from build123d import *

# Parameters (mm, degrees)
F1_DEPTH = 10
F3_START = -1.5
F3_DEPTH = 7
F4_R     = 5


with BuildPart() as f1:
    # F0 (on Top) → F1 (new body)
    with BuildSketch(Plane.XY):
        Polygon((0, 18.8854382), (-29.0617011202, 40), (-17.9611190632, 5.83592135), align=None)
        Polygon((17.9611190632, 5.83592135), (29.0617011202, 40), (0, 18.8854382), align=None)
        Polygon((0, 18.8854382), (-17.9611190632, 5.83592135), (-11.100582057, -15.27864045), (11.100582057, -15.27864045), (17.9611190632, 5.83592135), align=None)
        Polygon((11.100582057, -15.27864045), (47.0228201834, -15.27864045), (17.9611190632, 5.83592135), align=None)
        Polygon((-11.100582057, -15.27864045), (0, -49.4427191), (11.100582057, -15.27864045), align=None)
        Polygon((-17.9611190632, 5.83592135), (-47.0228201834, -15.27864045), (-11.100582057, -15.27864045), align=None)
    extrude(amount=F1_DEPTH)

    # F2 (on face) → F3 (cut)
    with BuildSketch(Plane.XY.offset(10).offset(F3_START)):
        Polygon((-9.25, -11.1145618), (0, -11.1145618), (9.25, -11.1145618), (9.25, 25.605956584), (0, 18.8854382), (-9.25, 25.605956584), align=None)
    extrude(amount=-F3_DEPTH, mode=Mode.SUBTRACT)

    # F4
    f4_edges = [f1.edges().sort_by_distance(p)[0] for p in [
        (-17.961119, 5.835921, 5),
        (-11.100582, -15.27864, 5),
        (11.100582, -15.27864, 5),
        (17.961119, 5.835921, 5),
        (0, 18.885438, 9.25),
        (0, 18.885438, 0.75),
        (9.25, 25.605957, 5),
        (-9.25, 25.605957, 5),
    ]]
    fillet(f4_edges, radius=F4_R)


solid = f1.part
Could you check a few things on this model? Use its own coordinates, in mm. A direction names the side the tool comes from. Give positions to 0.01 mm unless a question says otherwise; leave off trailing zeros. Order: outer loops, then holes, each group sorted by start corner. A loop starts at its lowest first (then second) coordinate and runs counter-clockwise, first axis right, second up. Notation, with made-up numbers: (-15, -37.5) -> (17, -37.5) arc R31 ccw to (17, -4.5) -> close; hole circle Ø9 at (28.25, 40.5). An arc over 180 degrees is marked (long way). Answer in a Markdown table with one row per item. Add a question column.
Item 1: Imagine slicing it at C-C (y = -10). List the corners of the cut face in (x, z) for me, and give its area (3 significant figures).
Item 2: Please list where these lines run through material, in increasing order: probe 1 along Z at (x, y) = (8.5, 10); probe 2 along X at (y, z) = (7, 3); probe 3 along X at (y, z) = (-3, 6).
Item 3: We'd pull the mould along Y, two halves only. Please class faces 6 (the flat face through (31, -15.279, 5)), 7 (the flat face through (3, -1, 10)), 8 (the flat face through (-33.779, -5.656, 4.93)): pulls with the +Y half, pulls with the -Y half, needs draft (parallel to the pull), parting line crosses it, or undercut.
Item 4: Imagine slicing it at A-A (x = -25.5). List the corners of the cut face in (y, z) for me, and give its area (3 significant figures).
Item 5: Imagine slicing it at D-D (x = -7). List the corners of the cut face in (y, z) for me, and give its area (3 significant figures).
Item 6: I'm going to push flat-ended pins straight in: P1, Ø5.5, axis at y = 4.5, z = 6.5, coming from the +X side; P2, Ø3, axis at x = 26.5, z = 7, coming from the -Y side; P3, Ø5, axis at x = 37.5, z = 3, coming from the +Y side. Where does each tip first touch, or does it pass through?
Item 7: For faces 1 (the flat face through (3, -1, 0)), 2 (the flat face through (-31, -15.279, 5)), 3 (the flat face through (19.086, 32.752, 4.93)), 4 (the flat face through (0, 4, 1.5)), 5 (the cylindrical face through (-19.07, 6.24, 5.07)), which set-ups out of +Z, -Z, +X, -X, +Y, -Y let a thin tool reach every point of the face, with its end or its side?
Item 8: Imagine slicing it at B-B (z = 3). List the corners of the cut face in (x, y) for me.
Result:
| question | item | result |
|---|---|---|
| 1 | outline | (-39.76, 0) -> (39.76, 0) -> (39.76, 10) -> (-39.76, 10) -> close; hole (-9.25, 1.5) -> (9.25, 1.5) -> (9.25, 8.5) -> (-9.25, 8.5) -> close |
| 1 | area | 666 mm2 |
| 2 | probe 1 | 0 to 1.5, 8.5 to 10 |
| 2 | probe 2 | -18.89 to -9.25, 9.25 to 18.89 |
| 2 | probe 3 | -30.12 to -9.25, 9.25 to 30.12 |
| 3 | face 6 | pulls with the -Y half |
| 3 | face 7 | needs draft |
| 3 | face 8 | undercut |
| 4 | outline | (-15.28, 0) -> (0.36, 0) -> (0.36, 10) -> (-15.28, 10) -> close; (29.04, 0) -> (37.41, 0) -> (37.41, 10) -> (29.04, 10) -> close |
| 4 | area | 240 mm2 |
| 5 | outline | (-27.9, 0) -> (23.97, 0) -> (23.97, 1.5) -> (-11.11, 1.5) -> (-11.11, 8.5) -> (23.97, 8.5) -> (23.97, 10) -> (-27.9, 10) -> close |
| 5 | area | 273 mm2 |
| 6 | P1 | x = 23.58 |
| 6 | P2 | y = -15.28 |
| 6 | P3 | y = -6.54 |
| 7 | face 1 | -Z, +X, -X, +Y, -Y |
| 7 | face 2 | +Z, -Z, -X, -Y |
| 7 | face 3 | +Z, -Z, +Y |
| 7 | face 4 | +Y |
| 7 | face 5 | +Z, -Z, -X |
| 8 | outline | (-47.02, -15.28) -> (-14.73, -15.28) arc R5 cw to (-9.98, -18.73) -> (0, -49.44) -> (9.98, -18.73) arc R5 cw to (14.73, -15.28) -> (47.02, -15.28) -> (20.9, 3.7) arc R5 cw to (19.08, 9.29) -> (29.06, 40) -> (11.31, 27.1) arc R5 ccw to (9.25, 23.06) -> (9.25, -11.11) -> (-9.25, -11.11) -> (-9.25, 23.06) arc R5 ccw to (-11.31, 27.1) -> (-29.06, 40) -> (-19.08, 9.29) arc R5 cw to (-20.9, 3.7) -> close |
